The listing builds one solid part. Answer for the finished solid, in the listing's coordinates (mm). A direction names the side the tool comes from. Round coordinates to 2 decimals unless told otherwise and drop trailing zeros. Loops run counter-clockwise (first coordinate to the right, second up) from the corner with the lowest first, then second, coordinate; pieces in that order, holes last. Notation, with made-up numbers: (45, 49) -> (93, 49) arc R22 ccw to (93, 87) -> close; hole circle Ø11 at (51.5, -39.5). An arc over 180 degrees is marked (long way). Answer in a Markdown table with one row per item. Add a question column.
Autodesk Inventor part; units mm, degrees
ref_plane "YZ Plane" through (0, 0, 0) normal (1, 0, 0) x (0, 1, 0)
ref_plane "XZ Plane" through (0, 0, 0) normal (0, 1, 0) x (-1, 0, 0)
ref_plane "XY Plane" through (0, 0, 0) normal (0, 0, 1) x (1, 0, 0)
sketch "Sketch1" plane through (0, 0, 0) normal (0, 1, 0) x (-1, 0, 0)
  line L0 (41.0588, -14.3587) -> (13.6765, -27.82)
  arc A0 (-13.6765, -27.82) -> (13.6765, -27.82) centre (0, 0) ccw
  line L1 (-13.6765, -27.82) -> (-41.0588, -14.3587)
  arc A1 (-41.0588, 14.3587) -> (-41.0588, -14.3587) centre (-34, 0) ccw
  line L2 (-41.0588, 14.3587) -> (-13.6765, 27.82)
  arc A2 (13.6765, 27.82) -> (-13.6765, 27.82) centre (0, 0) ccw
  line L3 (13.6765, 27.82) -> (41.0588, 14.3587)
  arc A3 (41.0588, -14.3587) -> (41.0588, 14.3587) centre (34, 0) ccw
  dimension "d0" = 68
  dimension "d1" = 16
  dimension "d2" = 31
extrude "Extrusion1" add sketch "Sketch1" along normal blind 15
sketch "Sketch2" plane through (0, 15, 0) normal (0, 1, 0) x (1, 0, 0)
  arc A0 (-13.6765, -27.82) -> (13.6765, -27.82) centre (0, 0) ccw
  circle A1 centre (0, 0) radius 20
  dimension "d5" = 40
extrude "Extrusion2" add sketch "Sketch2" along normal blind 27
fillet "Fillet1" radius 4 1 edges at (-20, 15, 0)
sketch "Sketch3" plane through (0, 0, 0) normal (0, 0, 1) x (1, 0, 0)
  line L0 (20, 42) -> (-20, 42)
  arc A0 (20, 42) -> (0, 62) centre (0, 42) ccw
  line L1 (0, -13.2284) -> (0, 79.3706)
  point P0 (0, 0)
  point P1 (0, 42)
revolve "Revolution1" add sketch "Sketch3" angle 360 about axis through (0, -10, 0) along (0, 1, 0)
sketch "Sketch4" plane through (0, 0, 0) normal (0, 0, 1) x (1, 0, 0)
  arc A0 (20, 42) -> (-20, 42) centre (0, 42) ccw
  arc A1 (20, 42) -> (-20, 42) centre (0, 42) ccw
  line L0 (10, 0) -> (10, 42)
  arc A2 (10, 42) -> (0, 52) centre (0, 42) ccw
  line L1 (0, -12.4) -> (0, 74.4)
  line L2 (10, 0) -> (0, 0)
  dimension "d10" = 20
revolve "Revolution2" cut sketch "Sketch4" angle 360 about axis through (0, -10, 0) along (0, 1, 0)
sketch "Sketch5" plane through (0, 0, 0) normal (0, 0, 1) x (1, 0, 0)
  arc A0 (10, 42) -> (-10, 42) centre (0, 42) ccw
  arc A1 (-6, 42) -> (6, 42) centre (0, 42) ccw
  line L0 (-6, 42) -> (-6, 61.0788)
  line L1 (6, 42) -> (6, 61.0788)
  line L2 (20, 42) -> (-20, 42)
  arc A2 (20, 42) -> (-20, 42) centre (0, 42) ccw
  arc A3 (6, 61.0788) -> (-6, 61.0788) centre (0, 42) ccw
  point P0 (0, 0)
  dimension "d12" = 6
extrude "Extrusion3" cut sketch "Sketch5" along normal through all both and the other way through all contours L1 L2 L0 A0 | A0 L0 A2 L1 | A1 L2
sketch "Sketch6" plane through (0, 0, 0) normal (1, 0, 0) x (0, 1, 0)
  arc A0 (42, -8) -> (42, 8) centre (42, 0) ccw
  circle A1 centre (42, 0) radius 5
  point P0 (0, 0)
  dimension "d15" = 10
extrude "Extrusion4" cut sketch "Sketch6" along normal through all both and the other way through all
sketch "Sketch7" plane through (0, 15, 0) normal (0, 1, 0) x (1, 0, 0)
  arc A0 (41.0588, -14.3587) -> (41.0588, 14.3587) centre (34, 0) ccw
  arc A1 (-41.0588, 14.3587) -> (-41.0588, -14.3587) centre (-34, 0) ccw
hole "Hole1" at (-34, 15, 0) at (34, 15, 0) direction (0, -1, 0) diameter 12 end through all
properties part number "Part010TiltSupport" material "Steel, Cast"
Item 1: Section D-D, the plane y = 57 is taken. Write down the section's boundary in (x, z).
Item 2: Flat-ended cylindrical pins translate along their axes: P1, Ø19, axis at x = 34, z = 0, coming from the -Y side; P2, Ø4, axis at y = 27.5, z = 14, coming from the +X side; P3, Ø12, axis at x = 36.5, z = 11, coming from the +Y side; P4, Ø16, axis at y = 42, z = 0, coming from the -X side. Find the tip coordinate at first contact, or state that the pin passes through.
Item 3: Section A-A, the plane x = 0 is taken. Write down the section's boundary in (y, z), and give its area (3 significant figures).
Item 4: Consider L1, parallel to X at y = 6, z = 0; L2, parallel to X at y = 21, z = 0. Determine where each line is inside the solid, lowest interval first. Write a range as from..to.
Item 5: Section B-B, the plane z = 0 is taken. Give the number of separate pieces and of enclosed holes in the cut face, and give its area (3 significant figures).
Item 6: For faces 4 (the flat face through (-27.18, 7.4, 21.18)), 5 (the cylindrical face through (18.475, 30.339, -7.66)), 6 (the cylindrical face through (-10, 21, 0)), 7 (the flat face through (27.559, 7.395, 20.995)), 8 (the flat face through (6, 51, 0)), determine the directions among +Z, -Z, +X, -X, +Y, -Y from which every point of the face is accessible in a straight line to the end or side of a thin tool.
Item 7: The mould has two halves that part along Y. Classify faces 1 (the cylindrical face through (0, 36, 14)), 2 (the cylindrical face through (-28.143, 7.395, -1.301)), 3 (the cylindrical face through (-14.251, 46.619, -1.915)): +Y half, -Y half, draft (parallel to the pull), parting line (faces both ways), or undercut.
Item 8: Section C-C, the plane y = 40 is taken. Write down the section's boundary in (x, z).
Here are the results:
| question | item | result |
|---|---|---|
| 1 | outline | (-6, -11.79) -> (-6, 11.79) arc R13.23 ccw to start; (6, -11.79) arc R13.23 ccw to (6, 11.79) -> close |
| 2 | P1 | stops at y = 0 |
| 2 | P2 | stops at x = 16 |
| 2 | P3 | stops at y = 15 |
| 2 | P4 | stops at x = -20 |
| 3 | outline | (0, -31) -> (15, -31) -> (15, -24) arc R4 cw to (19, -20) -> (36, -20) -> (36, -10) -> (0, -10) -> close; (0, 10) -> (36, 10) -> (36, 20) -> (19, 20) arc R4 cw to (15, 24) -> (15, 31) -> (0, 31) -> close |
| 3 | area | 1,060 mm² |
| 4 | L1 | x = -50..-40, -28..-10, 10..28, 40..50 |
| 4 | L2 | x = -20..-10, 10..20 |
| 5 | separate pieces | 6 |
| 5 | enclosed holes | 0 |
| 5 | area | 1,530 mm² |
| 6 | face 4 | +Z, -X, +Y, -Y |
| 6 | face 5 | +Y |
| 6 | face 6 | -Y |
| 6 | face 7 | +Z, +X, +Y, -Y |
| 6 | face 8 | +Z, -Z, +Y |
| 7 | face 1 | +Y half |
| 7 | face 2 | draft |
| 7 | face 3 | undercut |
| 8 | outline | (-19.47, -4.58) arc R20 ccw to (-5.66, -19.18) -> (-5.66, -8.25) arc R10 cw to (-8.89, -4.58) -> close; (-19.47, 4.58) -> (-8.89, 4.58) arc R10 cw to (-5.66, 8.25) -> (-5.66, 19.18) arc R20 ccw to start; (5.66, -19.18) arc R20 ccw to (19.47, -4.58) -> (8.89, -4.58) arc R10 cw to (5.66, -8.25) -> close; (5.66, 8.25) arc R10 cw to (8.89, 4.58) -> (19.47, 4.58) arc R20 ccw to (5.66, 19.18) -> close |
